Could you check a few things on this model? Use its own coordinates, in mm. A direction names the side the tool comes from. Coordinates: 2 decimals unless noted, no trailing zeros. Write each loop counter-clockwise with the first axis right and the second up, starting at its lowest first coordinate (ties: lowest second). Pieces come first, ordered by that corner, then holes.
```python
from build123d import *

# Parameters (mm, degrees)
F0_W     = 60
F0_H     = 60
F1_DEPTH = 2.5
F2_R     = 3.25
F3_DEPTH = 25
F4_R     = 15
F5_DEPTH = 0.8
F6_R     = 12
F7_DEPTH = 0.7
F7_TAPER = -50
F8_R     = 4.5
F9_DEPTH = 25
F10_R    = 5


with BuildPart() as f1:
    # F0 (on Top) → F1 (new body)
    with BuildSketch(Plane.XY):
        with Locations((22.8730514646, -21.4082733154)):
            Rectangle(F0_W, F0_H)
    extrude(amount=F1_DEPTH)

    # F2 (on face) → F3 (cut)
    with BuildSketch(Plane.XY.offset(2.5)):
        with Locations((0.3730514646, 1.0917266846)):
            Circle(F2_R)
        with Locations((45.3730514646, 1.0917266846)):
            Circle(F2_R)
        with Locations((45.3730514646, -43.9082733154)):
            Circle(F2_R)
        with Locations((0.3730514646, -43.9082733154)):
            Circle(F2_R)
    extrude(amount=-F3_DEPTH, mode=Mode.SUBTRACT)

    # F4 (on face) → F5 (cut)
    with BuildSketch(Plane.XY.offset(2.5)):
        with Locations((22.8730514646, -21.4082733154)):
            Circle(F4_R)
    extrude(amount=-F5_DEPTH, mode=Mode.SUBTRACT)

    # F6 (on face) → F7 (join)
    with BuildSketch(Plane.XY.offset(1.7)):
        with Locations((22.8730514646, -21.4082733154)):
            Circle(F6_R)
    extrude(amount=F7_DEPTH, taper=F7_TAPER)

    # F8 (on face) → F9 (cut)
    with BuildSketch(Plane.XY.offset(2.4)):
        with Locations((22.8730514646, -21.4082733154)):
            Circle(F8_R)
    extrude(amount=-F9_DEPTH, mode=Mode.SUBTRACT)

    # F10
    f10_edges = [f1.edges().sort_by_distance(p)[0] for p in [
        (-7.126949, -51.408273, 1.25),
        (52.873051, -51.408273, 1.25),
        (52.873051, 8.591727, 1.25),
        (-7.126949, 8.591727, 1.25),
    ]]
    fillet(f10_edges, radius=F10_R)


solid = f1.part
```
1. I want a section at A-A on y = 2. Please give me the cut outline in (x, z).
Verdict:
outline: (-7.13, 0) - (-2.75, 0) - (-2.75, 2.5) - (-7.13, 2.5) - close; (3.49, 0) - (42.25, 0) - (42.25, 2.5) - (3.49, 2.5) - close; (48.49, 0) - (52.87, 0) - (52.87, 2.5) - (48.49, 2.5) - close
2. I want a section at C-C on z = 0.65. Please give me the cut outline in (x, y), plus the area to 3 significant figures.
Verdict:
outline: (-7.13, -46.41) arc R5 ccw to (-2.13, -51.41) - (47.87, -51.41) arc R5 ccw to (52.87, -46.41) - (52.87, 3.59) arc R5 ccw to (47.87, 8.59) - (-2.13, 8.59) arc R5 ccw to (-7.13, 3.59) - close; hole circle Ø6.5 at (0.37, -43.91); hole circle Ø6.5 at (0.37, 1.09); hole circle Ø9 at (22.87, -21.41); hole circle Ø6.5 at (45.37, -43.91); hole circle Ø6.5 at (45.37, 1.09)
area: 3,380 mm2
3. For pin 1 (6 mm diameter, centred on x = 45.37, y = -43.91, fed in from -Z); pin 2 (13 mm diameter, centred on x = 28, y = -18.5, fed in from +Z), each with a flat end and sliding along its axis, tell me the tip position at first contact or that it passes through.
Verdict:
pin 1: passes through
pin 2: stops at z = 2.4
4. On a 3-axis mill with a long thin cutter (end or side, diameter ignored), from which of +Z, -Z, +X, -X, +Y, -Y can I reach the whole of each face in a straight line? I mean faces 1 (the face through (2.12, 3.83, 1.27)), 2 (the face through (7.888, -20.749, 2.106)), 3 (the face through (16, -11, 1.7)). Say none if no direction works.
Verdict:
face 1: +Z, -Z
face 2: +Z
face 3: none
5. I want a section at B-B on x = 9. Please give me the cut outline in (y, z).
Verdict:
outline: (-51.41, 0) - (8.59, 0) - (8.59, 2.5) - (-15.7, 2.5) - (-15.7, 1.7) - (-27.11, 1.7) - (-27.11, 2.5) - (-51.41, 2.5) - close
6. If we mould it in two halves opening along Y, with no side actions, what happens to faces 4 (the face through (28, -21, 2.4)), 5 (the face through (52.873, -22, 1)), 6 (the face through (-5.701, -49.905, 1.268))? For each: pulls with the +Y half, pulls with the -Y half, needs draft (parallel to the pull), parting line crosses it, or undercut.
Verdict:
face 4: undercut
face 5: needs draft
face 6: pulls with the -Y half
7. Please list where these lines run through material, in increasing order: line 1 along X through (y, z) = (3, 0.75); line 2 along Y through (x, z) = (47.5, 1.2); line 3 along Z through (x, y) = (22, -28.5).
Verdict:
line 1: x = -7.13 to -2.26, 3 to 42.74, 48 to 52.87
line 2: y = -51.41 to -46.37, -41.45 to -1.37, 3.55 to 8.59
line 3: z = 0 to 2.4
8. I want a section at D-D on y = -45.5. Please give me the cut outline in (x, z).
Verdict:
outline: (-7.13, 0) - (-2.46, 0) - (-2.46, 2.5) - (-7.13, 2.5) - close; (3.21, 0) - (42.54, 0) - (42.54, 2.5) - (3.21, 2.5) - close; (48.21, 0) - (52.87, 0) - (52.87, 2.5) - (48.21, 2.5) - close
